Read the model definition and answer for the solid it produces. Units are mm, in the model's axes. Give positions to 0.01 mm unless a question says otherwise; leave off trailing zeros. Write each loop counter-clockwise with the first axis right and the second up, starting at its lowest first coordinate (ties: lowest second). Pieces come first, ordered by that corner, then holes.
```python
from build123d import *

# Parameters (mm, degrees)
CHAMFER_SIZE = 1


with BuildPart() as part:
    # Sketch → Revolution (revolve)
    with BuildSketch(Plane.XY):
        Polygon((21.05, 51.7), (24.05, 51.7), (24.05, 26.7), (25.75, 25), (25.75, 0), (22.75, 0), (22.75, 25), (21.05, 26.7), align=None)
    revolve(axis=Axis((0, 0, 0), (0, 1, 0)))

    # Chamfer
    chamfer_edges = [part.edges().sort_by_distance(p)[0] for p in [
        (-24.05, 51.7, 0),
        (-22.75, 0, 0),
    ]]
    chamfer(chamfer_edges, length=CHAMFER_SIZE)


solid = part.part
```
Item 1: Section A-A (z = 0) is taken. Write down the section's boundary in (x, y), and give its area (3 significant figures).
Result set:
outline: (-25.75, 0) - (-23.75, 0) - (-22.75, 1) - (-22.75, 25) - (-21.05, 26.7) - (-21.05, 51.7) - (-23.05, 51.7) - (-24.05, 50.7) - (-24.05, 26.7) - (-25.75, 25) - close; (21.05, 26.7) - (22.75, 25) - (22.75, 1) - (23.75, 0) - (25.75, 0) - (25.75, 25) - (24.05, 26.7) - (24.05, 50.7) - (23.05, 51.7) - (21.05, 51.7) - close
area: 308 mm2
Item 2: Each of these flat-tipped pins is pushed along its axis until it touches: pin 1 Ø10 at (x, y) = (19, 42.5) entering from -Z; pin 2 Ø8 at (x, y) = (-14, 22) entering from -Z; pin 3 Ø3 at (x, y) = (-20.5, 28) entering from +Z; pin 4 Ø3 at (x, z) = (17.5, 10) entering from +Y. Where does it stop, or does it pass through?
Result set:
pin 1: stops at z = -19.56
pin 2: stops at z = -23.73
pin 3: stops at z = 14.74
pin 4: stops at y = 51.7
Item 3: Determine the mould class of faces 1 (the cylindrical face through (-18.054, 13.168, 13.843)), 2 (the flat face through (-10, 51.7, 19)), 3 (the cylindrical face through (-19.09, 38.53, 14.63)) for opening direction Z: pulls with the +Z half, pulls with the -Z half, needs draft (parallel to the pull), parting line crosses it, or undercut.
Result set:
face 1: undercut
face 2: needs draft
face 3: parting line crosses it
Item 4: Section B-B (x = 0) is taken. Write down the section's boundary in (y, z).
Result set:
outline: (0, -25.75) - (25, -25.75) - (26.7, -24.05) - (50.7, -24.05) - (51.7, -23.05) - (51.7, -21.05) - (26.7, -21.05) - (25, -22.75) - (1, -22.75) - (0, -23.75) - close; (0, 23.75) - (1, 22.75) - (25, 22.75) - (26.7, 21.05) - (51.7, 21.05) - (51.7, 23.05) - (50.7, 24.05) - (26.7, 24.05) - (25, 25.75) - (0, 25.75) - close
Item 5: Section C-C (y = 17.5) is taken. Write down the section's boundary in (x, z).
Result set:
outline: circle Ø51.5 at (0, 0); hole circle Ø45.5 at (0, 0)
Item 6: Find the intervals of material crossed by line 1 along X through (y, z) = (7, 0); line 2 along X through (y, z) = (44, 0), in increasing order.
Result set:
line 1: x = -25.75 to -22.75, 22.75 to 25.75
line 2: x = -24.05 to -21.05, 21.05 to 24.05
Item 7: Section D-D (y = 43) is taken. Write down the section's boundary in (x, z), and give its area (3 significant figures).
Result set:
outline: circle Ø48.1 at (0, 0); hole circle Ø42.1 at (0, 0)
area: 425 mm2
